```python
from build123d import *

# Parameters (mm, degrees)
SKETCH1_W                                      = 60
SKETCH1_H                                      = 50.1
SKETCH1_R                                      = 1.5
SKETCH1_R_2                                    = 0.5
BOSS_EXTRUDE2_DEPTH                            = 3.5
M3_CLEARANCE_HOLE1_D                           = 3.2
M3_CLEARANCE_HOLE1_DEPTH                       = 3.5
CSK_FOR_M4_FLAT_HEAD_MACHINE_SCREW1_AT_2_COUNT = 2
CSK_FOR_M4_FLAT_HEAD_MACHINE_SCREW1_AT_2_PITCH = 40


with BuildPart() as part:
    # Sketch1 → Boss-Extrude2 (new body)
    with BuildSketch(Plane(origin=(0, 0, 0), x_dir=(1, 0, 0), z_dir=(0, 1, 0))):
        Rectangle(SKETCH1_W, SKETCH1_H)
        with Locations((-24, 19.05)):
            Circle(SKETCH1_R, mode=Mode.SUBTRACT)
        with Locations((-24, -19.05)):
            Circle(SKETCH1_R, mode=Mode.SUBTRACT)
        with Locations((24, -19.05)):
            Circle(SKETCH1_R, mode=Mode.SUBTRACT)
        with Locations((24, 19.05)):
            Circle(SKETCH1_R, mode=Mode.SUBTRACT)
        with Locations((20, 0)):
            Circle(SKETCH1_R_2, mode=Mode.SUBTRACT)
        with Locations((-20, 0)):
            Circle(SKETCH1_R_2, mode=Mode.SUBTRACT)
    extrude(amount=BOSS_EXTRUDE2_DEPTH)

    # M3 Clearance Hole1
    with Locations(Plane(origin=(0, 3.5, 0), x_dir=(1, 0, 0), z_dir=(0, 1, 0))):
        with Locations((-24, 19.05), (24, 19.05), (24, -19.05), (-24, -19.05)):
            Hole(M3_CLEARANCE_HOLE1_D / 2, depth=M3_CLEARANCE_HOLE1_DEPTH)

    # Sketch5 → CSK for M4 Flat Head Machine Screw1 (revolve, cut)
    with BuildSketch(Plane(origin=(-20, 3.5, 0), x_dir=(0, 0, 1), z_dir=(1, 0, 0))):
        Polygon((0, 0), (0, 3.5), (2.15, 3.5), (2.15, 2.55), (4.7, 0), align=None)
    csk_for_m4_flat_head_machine_screw1 = revolve(axis=Axis((-20, 9.85, 0), (0, -1, 0)), mode=Mode.SUBTRACT)

    # CSK for M4 Flat Head Machine Screw1 at 2: CSK for M4 Flat Head Machine Screw1 ×2
    with Locations(*[(i * CSK_FOR_M4_FLAT_HEAD_MACHINE_SCREW1_AT_2_PITCH, 0, 0) for i in range(1, CSK_FOR_M4_FLAT_HEAD_MACHINE_SCREW1_AT_2_COUNT)]):
        add(csk_for_m4_flat_head_machine_screw1, mode=Mode.SUBTRACT)


solid = part.part
```
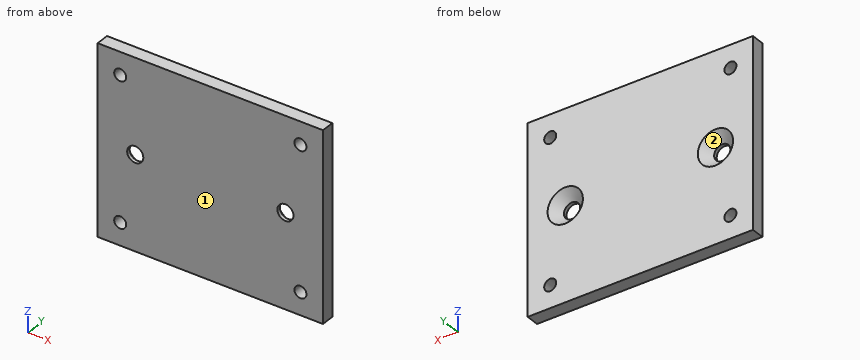
Check sheet for the modelled part. Datum: model origin and axes. Units: mm. Face numbers are marked on the shaded views. Coordinates: 2 decimals unless noted, no trailing zeros. Order: outer loops, then holes, each group sorted by start corner. A loop starts at its lowest first (then second) coordinate and runs counter-clockwise, first axis right, second up. Notation, with made-up numbers: M -5,77 L 27,77 A5 ccw 27,86 Z; hole C 56.25,6 d4. An arc over 180 degrees is marked long. Write each question's results on one line, items separated by ' | '. Start each with the question number.
1. Cross-section at B-B on x = 20. Record the cut outline in (y, z), and give its area (3 significant figures).
2. Mould release check, pull along X, two halves, no side actions. Record for the marked faces 1 and 2: +X half, -X half, draft (parallel to the pull), parting line (faces both ways), or undercut.
3. Go/stop test with flat-tipped pins: P1, Ø5, axis at x = -24, z = -19.05, coming from the -Y side; P2, Ø5.5, axis at x = -20, z = 0, coming from the +Y side; P3, Ø2.5, axis at x = 20, z = 0, coming from the -Y side (3 decimals). Record where each tip stops, or that it passes through.
4. Cross-section at A-A on z = 19.05. Record the cut outline in (x, y).
5. Cross-section at C-C on y = 1.75. Record the cut outline in (x, z), and give its area (3 significant figures).
6. Material ranges on probe 1 along X at (y, z) = (0.7, 0); probe 2 along Z at (x, y) = (-24, 1.6); probe 3 along X at (y, z) = (0.8, 19.05), recorded low to high.
Checks:
1) outline: M 0,-25.05 L 3.5,-25.05 L 3.5,-4.7 L 0.95,-2.15 L 0,-2.15 Z; M 0,2.15 L 0.95,2.15 L 3.5,4.7 L 3.5,25.05 L 0,25.05 Z | area: 154 mm²
2) face 1: draft | face 2: undercut
3) P1: stops at y = 0 | P2: stops at y = 1.55 | P3: passes through
4) outline: M -30,0 L -25.6,0 L -25.6,3.5 L -30,3.5 Z; M -22.4,0 L 22.4,0 L 22.4,3.5 L -22.4,3.5 Z; M 25.6,0 L 30,0 L 30,3.5 L 25.6,3.5 Z
5) outline: M -30,-25.05 L 30,-25.05 L 30,25.05 L -30,25.05 Z; hole C -24,-19.05 d3.2; hole C -24,19.05 d3.2; hole C -20,0 d5.9; hole C 20,0 d5.9; hole C 24,-19.05 d3.2; hole C 24,19.05 d3.2 | area: 2,920 mm²
6) probe 1: x = -30 to -22.15, -17.85 to 17.85, 22.15 to 30 | probe 2: z = -25.05 to -20.65, -17.45 to 17.45, 20.65 to 25.05 | probe 3: x = -30 to -25.6, -22.4 to 22.4, 25.6 to 30
